```python
from build123d import *

# Parameters (mm, degrees)
BOSS_EXTRUDE1_DEPTH = 19.05


with BuildPart() as part:
    # Sketch2 → Boss-Extrude1 (new body)
    with BuildSketch(Plane.ZY):
        Polygon((0, 0), (-933.45, 0), (-933.45, 914.4), (-463.55, 914.4), (0, 469.9), align=None)
    extrude(amount=BOSS_EXTRUDE1_DEPTH)


solid = part.part
```
For this review, take the finished solid that the model builds, in its own axes (mm). Round coordinates to 2 decimals unless told otherwise and drop trailing zeros. Write each loop counter-clockwise with the first axis right and the second up, starting at its lowest first coordinate (ties: lowest second). Pieces come first, ordered by that corner, then holes. Notation, with made-up numbers: (69, -6.5) - (90, -6.5) arc R15 cw to (90, 9.5) - close; hole circle Ø11 at (11.5, 3.25). An arc over 180 degrees is marked (long way). Answer as a JSON object with one key per item and string values.
1. We need section C-C on y = 670. Give the boundary of the cut face in (x, z), then the cut area to 3 significant figures.
Response values:
{"outline": "(-19.05, -933.45) - (0, -933.45) - (0, -208.68) - (-19.05, -208.68) - close", "area": "13,800 mm2"}
2. We need section B-B on z = -399. Give the boundary of the cut face in (x, y).
Response values:
{"outline": "(-19.05, 0) - (0, 0) - (0, 852.5) - (-19.05, 852.5) - close"}
3. To check wall thickness, follow line 1 along Z through (x, y) = (-10.5, 552); line 2 along Z through (x, y) = (-13.25, 667); line 3 along Y through (x, z) = (-12.75, -76). State the ranges of each line that lie inside material, in increasing order.
Response values:
{"line 1": "z = -933.45 to -85.62", "line 2": "z = -933.45 to -205.55", "line 3": "y = 0 to 542.78"}
4. We need section A-A on x = -14.25. Give the boundary of the cut face in (y, z), then the cut area to 3 significant figures.
Response values:
{"outline": "(0, -933.45) - (914.4, -933.45) - (914.4, -463.55) - (469.9, 0) - (0, 0) - close", "area": "751,000 mm2"}
5. For pin 1 Ø8 at (x, z) = (-6, -233) entering from +Y; pin 2 Ø2 at (x, y) = (-5.5, 641) entering from +Z, all flat-tipped, find the tip position at first contact; note any pin that passes through.
Response values:
{"pin 1": "stops at y = 697.16", "pin 2": "stops at z = -177.39"}
